Autodesk Inventor part; units mm, degrees
ref_plane "YZ Plane" through (0, 0, 0) normal (1, 0, 0) x (0, 1, 0)
ref_plane "XZ Plane" through (0, 0, 0) normal (0, 1, 0) x (-1, 0, 0)
ref_plane "XY Plane" through (0, 0, 0) normal (0, 0, 1) x (1, 0, 0)
sketch "Sketch1" plane through (0, 0, 0) normal (0, 0, 1) x (1, 0, 0)
  circle A0 centre (0, 0) radius 19.05
  dimension "d0" = 38.1
extrude "Extrusion1" add sketch "Sketch1" along normal blind 4.7752
sketch "Sketch2" plane through (0, 0, 0) normal (0, 0, -1) x (-1, 0, 0)
  circle A0 centre (0, 0) radius 19.05
  circle A1 centre (0, 0) radius 9.525
  dimension "d5" = 19.05
extrude "Extrusion2" add sketch "Sketch2" against normal blind 38.1 contours A1
sketch "Sketch3" plane through (0, 0, 0) normal (0, 0, -1) x (-1, 0, 0)
  circle A0 centre (0, 0) radius 19.05
  circle A1 centre (0, 14.2875) radius 2.5781
  dimension "d10" = 5.1562
  dimension "d12" = 14.2875
extrude "Extrusion3" cut sketch "Sketch3" against normal through all contours A1
pattern_circular "Circular Pattern1" count 3 over 360 about axis through (0, 0, 0) along (0, 0, 1) of "Extrusion3"
properties part number "LEAD NUT BLANK"
Check sheet for the modelled part. Datum: model origin and axes. Units: mm. A direction names the side the tool comes from. Give positions to 0.01 mm unless a question says otherwise; leave off trailing zeros. Loops run counter-clockwise (first coordinate to the right, second up) from the corner with the lowest first, then second, coordinate; pieces in that order, holes last. Notation, with made-up numbers: M -38,59.25 L -33,59.25 A33 cw -33,93.25 Z; hole C -33,79 d2. An arc over 180 degrees is marked long. Use a Markdown table: item, result. Add a question column.
Q1. Go/stop test with flat-tipped pins: pin 1 (1.5 mm diameter, centred on x = -13.5, y = 6, fed in from +Z); pin 2 (5 mm diameter, centred on y = 11, z = 32.5, fed in from +X); pin 3 (2 mm diameter, centred on y = 2.5, z = 19, fed in from +X); pin 4 (8 mm diameter, centred on x = 7.5, y = -8.5, fed in from +Z). Record where each tip stops, or that it passes through.
Q2. Tool access check on faces 1 (the flat face through (4, 9, 4.775)), 2 (the flat face through (0, 0, 38.1)). Record the directions out of +Z, -Z, +X, -X, +Y, -Y that give a thin tool (end or side, any length) a straight path to the whole face; none if there is none.
Q3. Sectioned sample at A-A, the plane x = 0. Record the cut outline in (y, z) (3 decimals).
Q4. Sectioned sample at D-D, the plane z = 2.5. Record the cut outline in (x, y).
Q5. Sectioned sample at B-B, the plane y = 0. Record the cut outline in (x, z) (3 decimals).
Q6. Mould release check, pull along Y, two halves, no side actions. Record for faces 3 (the flat face through (0, 0, 0)), 4 (the cylindrical face through (-11.81, -9.66, 2.35)), 5 (the cylindrical face through (7.559, -5.796, 21.204)): pulls with the +Y half, pulls with the -Y half, needs draft (parallel to the pull), parting line crosses it, or undercut.
Q7. Scan lines: line 1 along Y through (x, z) = (0, 2); line 2 along Z through (x, y) = (13.5, 11); line 3 along Y through (x, z) = (0.5, 17.5). Record each from-to range of solid material in increasing order. Write a range as [from, to].
Q8. Sectioned sample at C-C, the plane z = 24.5. Record the cut outline in (x, y) (3 decimals).
Verdict:
| question | item | result |
|---|---|---|
| 1 | pin 1 | z = 4.78 |
| 1 | pin 2 | x = 4.3 |
| 1 | pin 3 | x = 9.41 |
| 1 | pin 4 | z = 38.1 |
| 2 | face 1 | +Z |
| 2 | face 2 | +Z, +X, -X, +Y, -Y |
| 3 | outline | M -19.05,0 L 11.709,0 L 11.709,4.775 L 9.525,4.775 L 9.525,38.1 L -9.525,38.1 L -9.525,4.775 L -19.05,4.775 Z; M 16.866,0 L 19.05,0 L 19.05,4.775 L 16.866,4.775 Z |
| 4 | outline | C 0,0 d38.1; hole C -12.37,-7.14 d5.16; hole C 0,14.29 d5.16; hole C 12.37,-7.14 d5.16 |
| 5 | outline | M -19.05,0 L 19.05,0 L 19.05,4.775 L 9.525,4.775 L 9.525,38.1 L -9.525,38.1 L -9.525,4.775 L -19.05,4.775 Z |
| 6 | face 3 | needs draft |
| 6 | face 4 | undercut |
| 6 | face 5 | parting line crosses it |
| 7 | line 1 | [-19.05, 11.71], [16.87, 19.05] |
| 7 | line 2 | [0, 4.78] |
| 7 | line 3 | [-9.51, 9.51] |
| 8 | outline | C 0,0 d19.05 |
